Can you work these out from the drawing? Everything is in mm from the part's minimum corner. A direction names the side the tool comes from. Coordinates: 2 decimals unless noted, no trailing zeros. One line per question, with ' | ' between items. Start each with the question number.
1. Please list where these lines run through material, in increasing order: L1, parallel to Z at x = 57, y = 1 (1 decimal); L2, parallel to X at y = 63, z = 28.5 (1 decimal); L3, parallel to Z at x = 91, y = 88 (1 decimal). Write a range as [from, to].
2. We'd pull the mould along Z, two halves only. Please class the marked faces 3, 4 and 5: pulls with the +Z half, pulls with the -Z half, needs draft (parallel to the pull), parting line crosses it, or undercut.
3. Which directions (+Z, -Z, +X, -X, +Y, -Y) give clear straight access to the entire face, cutting with the end or side of a thin tool? Please do the marked faces 1 and 2.
4. I'm going to push flat-ended pins straight in: P1, Ø4, axis at x = 76, z = 7, coming from the +Y side (1 decimal); P2, Ø10.5, axis at x = 69.5, z = 12, coming from the +Y side (1 decimal). Where does each tip first touch, or does it pass through?
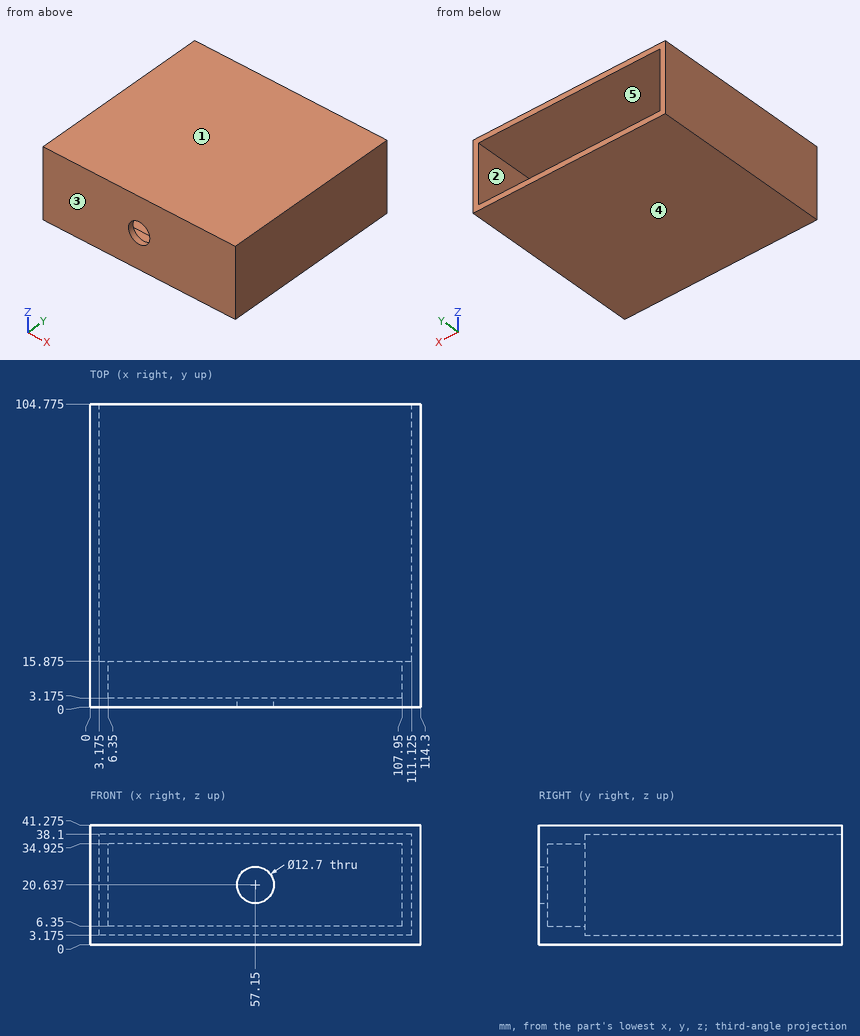
Results are:
1) L1: z = [0, 14.3], [27, 41.3] | L2: x = [0, 3.2], [111.1, 114.3] | L3: z = [0, 3.2], [38.1, 41.3]
2) face 3: needs draft | face 4: pulls with the -Z half | face 5: undercut
3) face 1: +Z, +X, -X, +Y, -Y | face 2: +Y
4) P1: stops at y = 15.9 | P2: stops at y = 3.2
